```python
from build123d import *

# Parameters (mm, degrees)
SKETCH1_W                       = 460
SKETCH1_H                       = 500
BOSS_EXTRUDE1_DEPTH             = 38.1
TAP_DRILL_FOR_M5X0_8_TAP1_D     = 4.2
TAP_DRILL_FOR_M5X0_8_TAP1_DEPTH = 20
TAP_DRILL_FOR_M5X0_8_TAP1_TIP   = 1.2618073
F_3_4_0_7500_DOWEL_HOLE1_D      = 19.05
SKETCH13_R                      = 90
CUT_EXTRUDE4_DEPTH              = 15
M14_CLEARANCE_HOLE1_D           = 15.5
TAP_DRILL_FOR_M10X1_5_TAP1_D    = 8.5
F_6_0MM_DOWEL_HOLE1_D           = 6
F_6_0MM_DOWEL_HOLE1_DEPTH       = 10
F_6_0MM_DOWEL_HOLE1_TIP         = 1.802581857


with BuildPart() as part:
    # Sketch1 → Boss-Extrude1 (new body)
    with BuildSketch(Plane(origin=(0, 0, 0), x_dir=(1, 0, 0), z_dir=(0, 1, 0))):
        Rectangle(SKETCH1_W, SKETCH1_H)
    extrude(amount=BOSS_EXTRUDE1_DEPTH)

    # Tap Drill for M5x0.8 Tap1
    with Locations(Plane(origin=(0, 38.1, 0), x_dir=(1, 0, 0), z_dir=(0, 1, 0))):
        with Locations((0, 65.786), (65.786, 0), (0, -65.786), (-65.786, 0)):
            Hole(TAP_DRILL_FOR_M5X0_8_TAP1_D / 2, depth=TAP_DRILL_FOR_M5X0_8_TAP1_DEPTH)
            with Locations((0, 0, -(TAP_DRILL_FOR_M5X0_8_TAP1_DEPTH + TAP_DRILL_FOR_M5X0_8_TAP1_TIP / 2))):  # 118° drill point
                Cone(0, TAP_DRILL_FOR_M5X0_8_TAP1_D / 2, TAP_DRILL_FOR_M5X0_8_TAP1_TIP, mode=Mode.SUBTRACT)

    # 3/4 (0.7500) Dowel Hole1 (through all)
    with Locations(Plane(origin=(0, 0, 0), x_dir=(-1, 0, 0), z_dir=(0, -1, 0))):
        with Locations((72.511608989, -30.035291873), (-30.035291873, -72.511608989), (30.035291873, 72.511608989), (-72.511608989, 30.035291873)):
            Hole(F_3_4_0_7500_DOWEL_HOLE1_D / 2)

    # Sketch13 → Cut-Extrude4 (cut)
    with BuildSketch(Plane.XZ):
        Circle(SKETCH13_R)
    extrude(amount=-CUT_EXTRUDE4_DEPTH, mode=Mode.SUBTRACT)

    # M14 Clearance Hole1 (through all)
    with Locations(Plane(origin=(0, 38.1, 0), x_dir=(1, 0, 0), z_dir=(0, 1, 0))):
        with Locations((66.67, -225.87), (-66.67, -225.87), (-66.67, 225.87), (66.67, 225.87)):
            Hole(M14_CLEARANCE_HOLE1_D / 2)

    # Tap Drill for M10x1.5 Tap1 (through all)
    with Locations(Plane(origin=(0, 0, 0), x_dir=(-1, 0, 0), z_dir=(0, -1, 0))):
        with Locations((178.438, 50.8), (203.838, 50.8), (178.438130466, -50.8), (203.838, -50.881410466)):
            Hole(TAP_DRILL_FOR_M10X1_5_TAP1_D / 2)

    # Ø6.0mm Dowel Hole1
    with Locations(Plane(origin=(0, 38.1, 0), x_dir=(1, 0, 0), z_dir=(0, 1, 0))):
        with Locations((-97.227182413, -97.227182413)):
            Hole(F_6_0MM_DOWEL_HOLE1_D / 2, depth=F_6_0MM_DOWEL_HOLE1_DEPTH)
            with Locations((0, 0, -(F_6_0MM_DOWEL_HOLE1_DEPTH + F_6_0MM_DOWEL_HOLE1_TIP / 2))):  # 118° drill point
                Cone(0, F_6_0MM_DOWEL_HOLE1_D / 2, F_6_0MM_DOWEL_HOLE1_TIP, mode=Mode.SUBTRACT)


solid = part.part
```
Geometry: final body of the model. Coordinates: model frame, mm. A direction names the side the tool comes from. Round coordinates to 2 decimals unless told otherwise and drop trailing zeros. Order: outer loops, then holes, each group sorted by start corner. A loop starts at its lowest first (then second) coordinate and runs counter-clockwise, first axis right, second up. Notation, with made-up numbers: (22, 75.5) -> (60, 75.5) arc R18 cw to (60, 81.5) -> close; hole circle Ø9 at (87, 60). An arc over 180 degrees is marked (long way). Use one line per item in the form item = value. Start each with the question number.
1. Cut plane A-A (z = -225.87). Return the cut outline in (x, y), then the cut area to 3 significant figures.
2. Pin query (flat end, axial travel): pin 1 Ø2.5 at (x, z) = (0, -65.786) entering from +Y; pin 2 Ø3.5 at (x, z) = (0, 65.786) entering from +Y. Return the tip coordinate at first contact, or that it passes through.
3. Reachability of faces 4 (the face through (-1, 15, 1)), 5 (the face through (-64.99, 18.783, 233.436)) from +Z, -Z, +X, -X, +Y, -Y: full face, straight path, thin tool, end or side. Return the list, or none.
4. Cut plane C-C (x = -28.5). Return the cut outline in (y, z).
5. Line query: probe 1 along Z at (x, y) = (0, 29); probe 2 along X at (y, z) = (19, -50.8); probe 3 along X at (y, z) = (24, 225). Output: solid intervals per line, ascending.
6. Cut plane B-B (y = 8.5). Count the separate pieces of the cut face and the enclosed holes in it, then the cut area to 3 significant figures.
7. Draft query along X for faces 1 (the face through (-65.661, 18.783, -233.554)), 2 (the face through (-3, 38.1, -4)), 3 (the face through (-230, 19, 3)). Return one class per face: pulls with the +X half, pulls with the -X half, needs draft (parallel to the pull), parting line crosses it, or undercut.
Solution:
q1.outline = (-230, 0) -> (-74.42, 0) -> (-74.42, 38.1) -> (-230, 38.1) -> close; (-58.92, 0) -> (58.92, 0) -> (58.92, 38.1) -> (-58.92, 38.1) -> close; (74.42, 0) -> (230, 0) -> (230, 38.1) -> (74.42, 38.1) -> close
q1.area = 16,300 mm^2
q2.pin_1 = 17.59
q2.pin_2 = 17.89
q3.face_4 = -Y
q3.face_5 = +Y, -Y
q4.outline = (0, -250) -> (38.1, -250) -> (38.1, -81.91) -> (15, -81.91) -> (15, -85.37) -> (0, -85.37) -> close; (0, 85.37) -> (15, 85.37) -> (15, -63.11) -> (38.1, -63.11) -> (38.1, 250) -> (0, 250) -> close
q5.probe_1 = -250 to -67.89, -63.69 to 63.69, 67.89 to 250
q5.probe_2 = -230 to -208.09, -199.59 to -182.69, -174.19 to 230
q5.probe_3 = -230 to -74.37, -58.97 to 58.97, 74.37 to 230
q6.separate_pieces = 1
q6.enclosed_holes = 9
q6.area = 204,000 mm^2
q7.face_1 = undercut
q7.face_2 = needs draft
q7.face_3 = pulls with the -X half
